from build123d import *

# Parameters (mm, degrees)
BOSS_EXTRUDE1_START = 8
SKETCH1_R           = 8
BOSS_EXTRUDE1_DEPTH = 6.333
SKETCH3_W           = 5.1
SKETCH3_H           = 5.1
CUT_EXTRUDE4_DEPTH  = 9


with BuildPart() as part:
    # Sketch1 → Boss-Extrude1 (new body)
    with BuildSketch(Plane.XY.offset(BOSS_EXTRUDE1_START)):
        Circle(SKETCH1_R)
    extrude(amount=-BOSS_EXTRUDE1_DEPTH)

    # Sketch3 → Cut-Extrude4 (cut, through all)
    with BuildSketch(Plane.XY):
        Rectangle(SKETCH3_W, SKETCH3_H)
    extrude(amount=CUT_EXTRUDE4_DEPTH, mode=Mode.SUBTRACT)


solid = part.part
Here's how the part is built. I have some questions about the finished solid (model axes, mm). A direction names the side the tool comes from. Round coordinates to 2 decimals unless told otherwise and drop trailing zeros. Order: outer loops, then holes, each group sorted by start corner. A loop starts at its lowest first (then second) coordinate and runs counter-clockwise, first axis right, second up. Notation, with made-up numbers: (-28.75, -22) -> (1.25, -22) arc R18 ccw to (1.25, -3) -> close; hole circle Ø7 at (-18.5, 11). An arc over 180 degrees is marked (long way). Use CSV: the item, a comma, the result in double quotes.
1. I want a section at D-D on y = -3.5. List the corners of the cut face in (x, z) for me, and give its area (3 significant figures).
Recorded:
outline,"(-7.19, 1.67) -> (7.19, 1.67) -> (7.19, 8) -> (-7.19, 8) -> close"
area,"91.1 mm2"
2. Which directions (+Z, -Z, +X, -X, +Y, -Y) give clear straight access to the entire face, cutting with the end or side of a thin tool? Please do faces 1 (the face through (0, 2.55, 5)), 2 (the face through (3, 0, 8)).
Recorded:
face 1,"+Z, -Z"
face 2,"+Z, +X, -X, +Y, -Y"
3. Thinking about a two-plate mould opening in X: for faces 3 (the face through (-1.73, -7.81, 4.88)), 4 (the face through (3, 0, 1.667)), 5 (the face through (0, -2.55, 5)), which applies, pulls with the +X half, pulls with the -X half, needs draft (parallel to the pull), parting line crosses it, or undercut?
Recorded:
face 3,"parting line crosses it"
face 4,"needs draft"
face 5,"undercut"
4. I need wall thicknesses on line 1 along Y through (x, z) = (1.25, 5.75); line 2 along X through (y, z) = (-1, 6); line 3 along Y through (x, z) = (-2.5, 7). Which ranges of each line are inside material? Lowest first, please.
Recorded:
line 1,"y = -7.9 to -2.55, 2.55 to 7.9"
line 2,"x = -7.94 to -2.55, 2.55 to 7.94"
line 3,"y = -7.6 to -2.55, 2.55 to 7.6"
5. I'm going to push flat-ended pins straight in: P1, Ø3, axis at x = -1, z = 2.5, coming from the -Y side; P2, Ø3, axis at x = 3.5, z = 3, coming from the +Y side; P3, Ø3, axis at y = 6.5, z = 2.5, coming from the +X side (3 decimals); P4, Ø1.5, axis at x = 1, z = 5.5, coming from the +Y side. Where does each tip first touch, or does it pass through?
Recorded:
P1,"stops at y = -8"
P2,"stops at y = 7.75"
P3,"stops at x = 6.245"
P4,"stops at y = 8"
6. I want a section at C-C on z = 5.5. List the corners of the cut face in (x, y) for me.
Recorded:
outline,"circle Ø16 at (0, 0); hole (-2.55, -2.55) -> (2.55, -2.55) -> (2.55, 2.55) -> (-2.55, 2.55) -> close"
7. I want a section at A-A on y = 0. List the corners of the cut face in (x, z) for me.
Recorded:
outline,"(-8, 1.67) -> (-2.55, 1.67) -> (-2.55, 8) -> (-8, 8) -> close; (2.55, 1.67) -> (8, 1.67) -> (8, 8) -> (2.55, 8) -> close"
